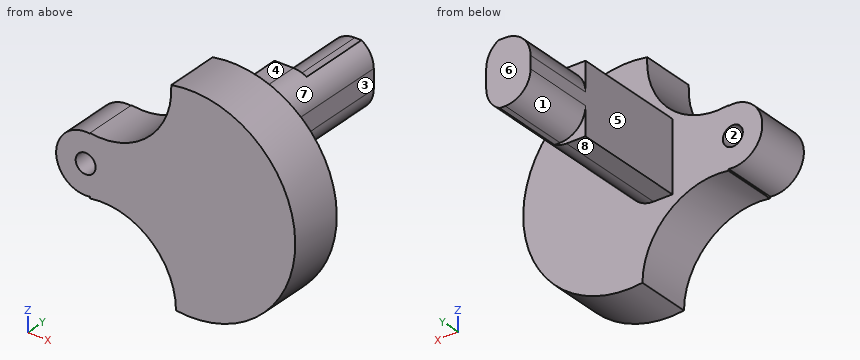
from build123d import *

# Parameters (mm, degrees)
F0_R     = 1.9939
F1_DEPTH = 10.9982
F2_W     = 14.542134
F2_H     = 12.6746
F3_DEPTH = 8.89
F4_R     = 5.08


with BuildPart() as f1:
    # F0 (on Front) → F1 (new body)
    with BuildSketch(Plane.XZ):
        with BuildLine():
            ThreePointArc((-20.13472, 5.986373), (-20.155318, 5.916654), (-20.175674, 5.846864))
            ThreePointArc((-20.175674, 5.846864), (-26.9113, 0), (-20.175674, -5.846864))
            ThreePointArc((-20.175674, -5.846864), (-20.133047, -5.992), (-20.089376, -6.136825))
            ThreePointArc((-20.089376, -6.136825), (-8.126305, -9.529423), (-2.886791, -20.806491))
            ThreePointArc((-2.886791, -20.806491), (21.000248, 0.482945), (-3.840213, 20.651789))
            ThreePointArc((-3.840213, 20.651789), (-8.446323, 9.384574), (-20.13472, 5.986373))
        make_face()
        with Locations((-21.0058, 0)):
            Circle(F0_R, mode=Mode.SUBTRACT)
    extrude(amount=F1_DEPTH)

    # F2 (on Right) → F3 (join)
    with BuildSketch(Plane.YZ):
        Polygon((0, 7.435056), (0, -6.560344), (23.0124, -6.560344), (23.0124, -5.96783), (23.0124, 6.70677), (23.0124, 7.435056), align=None)
        with Locations((30.283467, 0.36947)):
            Rectangle(F2_W, F2_H)
    extrude(amount=-F3_DEPTH)

    # F4
    f4_edges = [f1.edges().sort_by_distance(p)[0] for p in [
        (0, 11.5062, 7.435056),
        (0, 11.5062, -6.560344),
        (-8.89, 30.283467, 6.70677),
        (-8.89, 30.283467, -5.96783),
    ]]
    fillet(f4_edges, radius=F4_R)


solid = f1.part
Geometry check sheet. Reference: the model listing, model coordinates, mm. Face numbers are marked on the shaded views. A direction names the side the tool comes from. Round coordinates to 2 decimals unless told otherwise and drop trailing zeros. Order: outer loops, then holes, each group sorted by start corner. A loop starts at its lowest first (then second) coordinate and runs counter-clockwise, first axis right, second up. Notation, with made-up numbers: M 23.5,77 L 62.5,77 A25 ccw 62.5,102 Z; hole C -16.5,-36.75 d9. An arc over 180 degrees is marked long. Answer in a Markdown table with one row per item. Add a question column.
Item 1: Material ranges on L1, parallel to Y at x = 12, z = 4.5; L2, parallel to Z at x = -8, y = 12; L3, parallel to Z at x = -2.5, y = 23.5, recorded low to high. Write a range as [from, to].
Item 2: Sectioned sample at D-D, the plane y = 6. Enter the section's corners in (x, z), plus the area to 3 significant figures.
Item 3: Sectioned sample at A-A, the plane x = -21. Enter the section's corners in (y, z).
Item 4: Sectioned sample at B-B, the plane y = -5. Enter the section's corners in (x, z), plus the area to 3 significant figures.
Item 5: Depth check by flat-ended pin: pin 1 Ø12 at (y, z) = (19, 6) entering from +X; pin 2 Ø3 at (x, y) = (-7.5, 16) entering from -Z; pin 3 Ø5 at (x, y) = (-20, 0) entering from -Z. Enter the tip coordinate at first touch or a pass-through.
Item 6: Sectioned sample at C-C, the plane z = 0. Enter the section's corners in (x, y).
Item 7: Set-up check for the marked faces 5, 6, 7 and 8: record each of +Z, -Z, +X, -X, +Y, -Y from which the full face is reachable in a straight line by a thin tool's end or side.
Item 8: Draft check along Z on the marked faces 1, 2, 3 and 4. Enter one of: released by +Z, released by -Z, zero draft, split by the parting line, or undercut.
Filled in:
| question | item | result |
|---|---|---|
| 1 | L1 | y = [-11, 0] |
| 1 | L2 | z = [-6.56, 7.44] |
| 1 | L3 | z = [-5.86, 6.71] |
| 2 | outline | M -8.89,-6.56 L -5.08,-6.56 A5.08 ccw 0,-1.48 L 0,2.36 A5.08 ccw -5.08,7.44 L -8.89,7.44 Z |
| 2 | area | 113 mm² |
| 3 | outline | M -11,-5.91 L 0,-5.91 L 0,-1.99 L -11,-1.99 Z; M -11,1.99 L 0,1.99 L 0,5.91 L -11,5.91 Z |
| 4 | outline | M -20.18,-5.85 A21 ccw -20.09,-6.14 A14.92 cw -2.89,-20.81 A21.01 ccw long -3.84,20.65 A14 cw -20.13,5.99 A20.96 ccw -20.18,5.85 A5.91 ccw long Z; hole C -21.01,0 d3.99 |
| 4 | area | 1,170 mm² |
| 5 | pin 1 | stops at x = 0 |
| 5 | pin 2 | stops at z = -6.56 |
| 5 | pin 3 | stops at z = -6.14 |
| 6 | outline | M -26.91,-11 L -23,-11 L -23,0 L -26.91,0 Z; M -19.01,-11 L 21.01,-11 L 21.01,0 L 0,0 L 0,37.55 L -8.89,37.55 L -8.89,0 L -19.01,0 Z |
| 7 | face 5 | +Z, -Z, -X, +Y |
| 7 | face 6 | +Z, -Z, +X, -X, +Y |
| 7 | face 7 | +Z, +X, +Y |
| 7 | face 8 | -Z, +X, -X, +Y |
| 8 | face 1 | released by -Z |
| 8 | face 2 | undercut |
| 8 | face 3 | zero draft |
| 8 | face 4 | released by +Z |
